Could you check a few things on this model? Use its own coordinates, in mm. Face numbers are marked on the shaded views. Give positions to 0.01 mm unless a question says otherwise; leave off trailing zeros. Write each loop counter-clockwise with the first axis right and the second up, starting at its lowest first coordinate (ties: lowest second). Pieces come first, ordered by that corner, then holes. Notation, with made-up numbers: (44.5, 53.25) - (74.5, 53.25) arc R30 ccw to (74.5, 84.25) - close; hole circle Ø4 at (-27, -3.5). An arc over 180 degrees is marked (long way). Use one line per item in the form item = value.
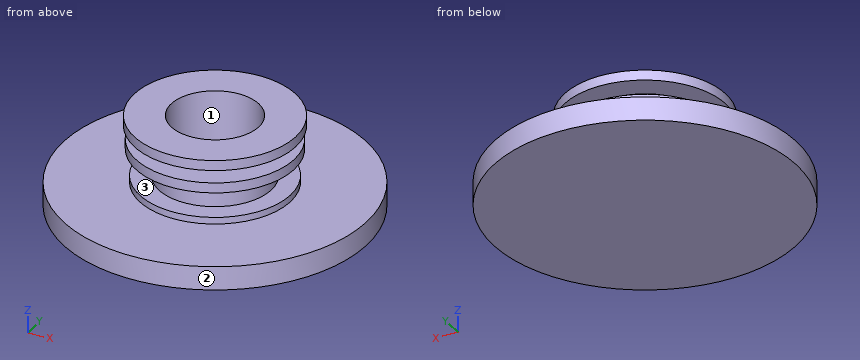
```python
from build123d import *

# Parameters (mm, degrees)
F0_R      = 22.5
F1_DEPTH  = 3.5
F2_R      = 11.2
F3_DEPTH  = 1
F4_R      = 8.35
F5_DEPTH  = 4
F6_R      = 11.75
F7_DEPTH  = 1.5
F8_R      = 8.35
F9_DEPTH  = 2
F10_R     = 12
F11_DEPTH = 1.5
F12_R     = 6.5
F13_DEPTH = 10


with BuildPart() as f1:
    # F0 (on Top) → F1 (new body)
    with BuildSketch(Plane.XY):
        Circle(F0_R)
    extrude(amount=F1_DEPTH)

    # F2 (on face) → F3 (join)
    with BuildSketch(Plane.XY.offset(3.5)):
        Circle(F2_R)
    extrude(amount=F3_DEPTH)

    # F4 (on face) → F5 (join)
    with BuildSketch(Plane.XY.offset(4.5)):
        Circle(F4_R)
    extrude(amount=F5_DEPTH)

    # F6 (on face) → F7 (join)
    with BuildSketch(Plane.XY.offset(8.5)):
        Circle(F6_R)
    extrude(amount=F7_DEPTH)

    # F8 (on face) → F9 (join)
    with BuildSketch(Plane.XY.offset(10)):
        Circle(F8_R)
    extrude(amount=F9_DEPTH)

    # F10 (on face) → F11 (join)
    with BuildSketch(Plane.XY.offset(12)):
        Circle(F10_R)
    extrude(amount=F11_DEPTH)

    # F12 (on face) → F13 (cut, through all)
    with BuildSketch(Plane.XY.offset(13.5)):
        Circle(F12_R)
    extrude(amount=-F13_DEPTH, mode=Mode.SUBTRACT)


solid = f1.part
```
1. For pin 1 (3 mm diameter, centred on x = -5.5, z = 4.5, fed in from -Y); pin 2 (8 mm diameter, centred on x = -4, z = 9, fed in from +Y); pin 3 (8 mm diameter, centred on y = -13.5, z = 6, fed in from +X), each with a flat end and sliding along its axis, tell me the tip position at first contact or that it passes through.
Response values:
pin_1 = -22.07
pin_2 = 11.92
pin_3 = 19.96
2. Imagine slicing it at D-D, the plane y = 17.5. List the corners of the cut face in (x, z) for me, and give its area (3 significant figures).
Response values:
outline = (-14.14, 0) - (14.14, 0) - (14.14, 3.5) - (-14.14, 3.5) - close
area = 99.0 mm²
3. If we mould it in two halves opening along Y, with no side actions, what happens to the marked faces 1, 2 and 3? For each: pulls with the +Y half, pulls with the -Y half, needs draft (parallel to the pull), parting line crosses it, or undercut.
Response values:
face_1 = undercut
face_2 = parting line crosses it
face_3 = needs draft
4. Imagine slicing it at A-A, the plane x = 0. List the corners of the cut face in (y, z) for me.
Response values:
outline = (-22.5, 0) - (22.5, 0) - (22.5, 3.5) - (11.2, 3.5) - (11.2, 4.5) - (8.35, 4.5) - (8.35, 8.5) - (11.75, 8.5) - (11.75, 10) - (8.35, 10) - (8.35, 12) - (12, 12) - (12, 13.5) - (6.5, 13.5) - (6.5, 3.5) - (-6.5, 3.5) - (-6.5, 13.5) - (-12, 13.5) - (-12, 12) - (-8.35, 12) - (-8.35, 10) - (-11.75, 10) - (-11.75, 8.5) - (-8.35, 8.5) - (-8.35, 4.5) - (-11.2, 4.5) - (-11.2, 3.5) - (-22.5, 3.5) - close
5. Imagine slicing it at C-C, the plane z = 1.5. List the corners of the cut face in (x, y) for me, and give its area (3 significant figures).
Response values:
outline = circle Ø45 at (0, 0)
area = 1,590 mm²
6. If I drill on line 1 (Z direction, x = -8.5, y = 6); line 2 (Y direction, x = 0, z = 8.75); line 3 (Z direction, x = -15.5, y = -8), over which ranges is the centre line in solid material (lowest first)? Write a range as from..to.
Response values:
line_1 = 0..4.5, 8.5..10, 12..13.5
line_2 = -11.75..-6.5, 6.5..11.75
line_3 = 0..3.5
